```python
from build123d import *

# Parameters (mm, degrees)
SKETCH1_W           = 270.887813212
SKETCH1_H           = 258.221174697
BASE_DEPTH          = 6
SKETCH2_W           = 6.892214754
SKETCH2_H           = 258.221174697
BOSS_EXTRUDE2_DEPTH = 80
FILLET1_R           = 5


with BuildPart() as part:
    # Sketch1 → Base (new body)
    with BuildSketch(Plane(origin=(0, 0, 0), x_dir=(1, 0, 0), z_dir=(0, 1, 0))):
        with Locations((-126.688596317, -107.886320424)):
            Rectangle(SKETCH1_W, SKETCH1_H)
    extrude(amount=BASE_DEPTH)

    # Sketch2 → Boss-Extrude2 (add)
    with BuildSketch(Plane(origin=(0, 6, 0), x_dir=(1, 0, 0), z_dir=(0, 1, 0))):
        with Locations((-258.686395546, -107.886320424)):
            Rectangle(SKETCH2_W, SKETCH2_H)
    extrude(amount=BOSS_EXTRUDE2_DEPTH)

    # Fillet1
    fillet1_edges = [part.edges().sort_by_distance(p)[0] for p in [
        (-255.240288169, 6, 107.886320423),
    ]]
    fillet(fillet1_edges, radius=FILLET1_R)


solid = part.part
```
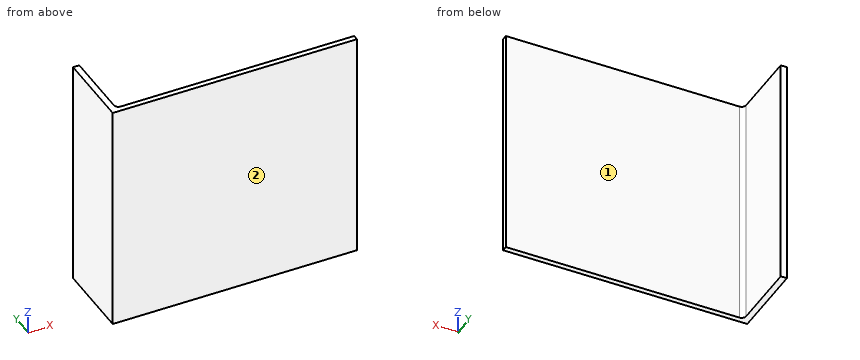
The listing builds one solid part. Answer for the finished solid, in the listing's coordinates (mm). Face numbers are marked on the shaded views. A direction names the side the tool comes from. Round coordinates to 2 decimals unless told otherwise and drop trailing zeros. Order: outer loops, then holes, each group sorted by start corner. A loop starts at its lowest first (then second) coordinate and runs counter-clockwise, first axis right, second up. Notation, with made-up numbers: (79, -31) -> (105, -31) arc R19 ccw to (105, -11) -> close; hole circle Ø3 at (77, 83.25). An arc over 180 degrees is marked (long way). Answer as CSV lines item,"result".
Q1. A cutting plane is placed at B-B on x = -83. Determine the outline of the cut face in (y, z).
Computed values:
outline,"(0, -21.22) -> (6, -21.22) -> (6, 237) -> (0, 237) -> close"
Q2. Consider line 1 (X direction, y = 58, z = 194.5); line 2 (Y direction, x = -3, z = 46); line 3 (X direction, y = 8.5, z = 119). Determine where each line is inside the solid, lowest interval first. Write a range as from..to.
Computed values:
line 1,"x = -262.13..-255.24"
line 2,"y = 0..6"
line 3,"x = -262.13..-254.57"
Q3. Which of the six approach directions +Z, -Z, +X, -X, +Y, -Y give full straight-line access (tool end or side, diameter ignored) to the marked faces 1 and 2?
Computed values:
face 1,"+Z, -Z, +X, +Y"
face 2,"+Z, -Z, +X, -X, -Y"
Q4. A cutting plane is placed at A-A on z = 132. Determine the outline of the cut face in (x, y).
Computed values:
outline,"(-262.13, 0) -> (8.76, 0) -> (8.76, 6) -> (-250.24, 6) arc R5 cw to (-255.24, 11) -> (-255.24, 86) -> (-262.13, 86) -> close"
Q5. Given pin 1 (12 mm diameter, centred on x = -135.5, z = 118.5, fed in from +Y); pin 2 (1 mm diameter, centred on y = 37, z = 7.5, fed in from +X), each flat-ended and moving along its own axis, determine where each tip first touches the part or whether it passes through.
Computed values:
pin 1,"stops at y = 6"
pin 2,"stops at x = -255.24"
Q6. A cutting plane is placed at C-C on y = 73. Determine the outline of the cut face in (x, z).
Computed values:
outline,"(-262.13, -21.22) -> (-255.24, -21.22) -> (-255.24, 237) -> (-262.13, 237) -> close"
